Verification items for the finished model (mm, model axes). A direction names the side the tool comes from. Give positions to 0.01 mm unless a question says otherwise; leave off trailing zeros. Loops run counter-clockwise (first coordinate to the right, second up) from the corner with the lowest first, then second, coordinate; pieces in that order, holes last. Notation, with made-up numbers: M 4,38 L 45,38 A25 ccw 45,52 Z; hole C -3.75,42 d4. An arc over 180 degrees is marked long. Use CSV: the item, a comma, the result in double quotes.
from build123d import *

# Parameters (mm, degrees)
F0_W     = 152.4
F0_H     = 152.4
F1_DEPTH = 3.175


with BuildPart() as f1:
    # F0 (on Top) → F1 (new body)
    with BuildSketch(Plane.XY):
        Rectangle(F0_W, F0_H)
        Polygon((-38.028175, -36.692278), (-33.612002, -23.464767), (-24.494429, -34.536101), (-13.657085, -25.611226), (0, -42.194824), (16.270282, -28.795762), (23.419121, -37.476491), (38.59369, -24.979782), (44.050138, -49.352157), (25.000943, -42.676793), (0, -52.934063), (-12.283398, -52.934063), (-19.935643, -43.002425), (-28.237687, -49.399082), align=None, mode=Mode.SUBTRACT)
        Polygon((-39.728351, 35.782534), (-37.243412, 41.580727), (-9.90904, 28.824696), align=None, mode=Mode.SUBTRACT)
        Polygon((39.728351, 35.782534), (9.90904, 28.824696), (37.243412, 41.580727), align=None, mode=Mode.SUBTRACT)
    extrude(amount=F1_DEPTH)


solid = f1.part
(1) Section check B-B on z = 1.75. Record the cut outline in (x, y), plus the area to 3 significant figures.
Calculated:
outline,"M -76.2,-76.2 L 76.2,-76.2 L 76.2,76.2 L -76.2,76.2 Z; hole M -39.73,35.78 L -9.91,28.82 L -37.24,41.58 Z; hole M -38.03,-36.69 L -28.24,-49.4 L -19.94,-43 L -12.28,-52.93 L 0,-52.93 L 25,-42.68 L 44.05,-49.35 L 38.59,-24.98 L 23.42,-37.48 L 16.27,-28.8 L 0,-42.19 L -13.66,-25.61 L -24.49,-34.54 L -33.61,-23.46 Z; hole M 9.91,28.82 L 39.73,35.78 L 37.24,41.58 Z"
area,"21,800 mm²"
(2) Section check A-A on x = 14. Record the cut outline in (y, z) (3 decimals), plus the area to 3 significant figures.
Calculated:
outline,"M -76.2,0 L -47.19,0 L -47.19,3.175 L -76.2,3.175 Z; M -30.665,0 L 29.779,0 L 29.779,3.175 L -30.665,3.175 Z; M 30.734,0 L 76.2,0 L 76.2,3.175 L 30.734,3.175 Z"
area,"428 mm²"
(3) Mould release check, pull along X, two halves, no side actions. Record for faces 3 (the flat face through (-16.056, -48.038, 1.565)), 4 (the flat face through (-1, 1, 3.175)): released by +X, released by -X, zero draft, split by the parting line, or undercut.
Calculated:
face 3,"undercut"
face 4,"zero draft"
(4) Section check C-C on x = -30.5. Record the cut outline in (y, z) (3 decimals), plus the area to 3 significant figures.
Calculated:
outline,"M -76.2,0 L -46.463,0 L -46.463,3.175 L -76.2,3.175 Z; M -27.244,0 L 33.629,0 L 33.629,3.175 L -27.244,3.175 Z; M 38.434,0 L 76.2,0 L 76.2,3.175 L 38.434,3.175 Z"
area,"408 mm²"
(5) Depth check by flat-ended pin: pin 1 Ø8 at (x, y) = (-24, 27) entering from -Z. Enter the tip coordinate at first touch or a pass-through.
Calculated:
pin 1,"stops at z = 0"
(6) Scan lines: L1, parallel to Y at x = -31, z = 2.75; L2, parallel to Y at x = -24, z = 2.65; L3, parallel to X at y = -30.5, z = 2.75. Record each from-to range of solid material in increasing order. Write a range as from..to.
Calculated:
L1,"y = -76.2..-45.81, -26.64..33.75, 38.67..76.2"
L2,"y = -76.2..-46.13, -34.13..32.11, 35.4..76.2"
L3,"x = -76.2..-35.96, -27.82..-19.59, -9.63..14.2, 17.67..31.89, 39.83..76.2"
(7) Tool access check on faces 1 (the flat face through (-1, 1, 0)), 2 (the flat face through (-6.92, -33.79, 1.57)). Record the directions out of +Z, -Z, +X, -X, +Y, -Y that give a thin tool (end or side, any length) a straight path to the whole face; none if there is none.
Calculated:
face 1,"-Z, +X, -X, +Y, -Y"
face 2,"+Z, -Z"
